from build123d import *

# Parameters (mm, degrees)
SCHIZZO1_R                   = 4.25
SCHIZZO1_R_2                 = 2.75
ESTRUSIONE_ESTRUSIONE1_DEPTH = 2.8
SCHIZZO2_R                   = 4.25
ESTRUSIONE_ESTRUSIONE2_DEPTH = 1
RACCORDO1_R                  = 2


with BuildPart() as part:
    # Schizzo1 → Estrusione-Estrusione1 (new body)
    with BuildSketch(Plane.XY):
        Circle(SCHIZZO1_R)
        Circle(SCHIZZO1_R_2, mode=Mode.SUBTRACT)
    extrude(amount=ESTRUSIONE_ESTRUSIONE1_DEPTH)

    # Schizzo2 → Estrusione-Estrusione2 (add)
    with BuildSketch(Plane.XY.offset(2.8)):
        Circle(SCHIZZO2_R)
    extrude(amount=ESTRUSIONE_ESTRUSIONE2_DEPTH)

    # Raccordo1
    raccordo1_edges = [part.edges().sort_by_distance(p)[0] for p in [
        (-4.25, 0, 3.8),
    ]]
    fillet(raccordo1_edges, radius=RACCORDO1_R)


solid = part.part
Can you work these out from the model? Positions are in its coordinate system, mm. A direction names the side the tool comes from. Coordinates: 2 decimals unless noted, no trailing zeros. Loops run counter-clockwise (first coordinate to the right, second up) from the corner with the lowest first, then second, coordinate; pieces in that order, holes last. Notation, with made-up numbers: (-1.5, 69.5) - (14.5, 69.5) arc R20 ccw to (14.5, 101.5) - close; hole circle Ø7 at (27, -15.5). An arc over 180 degrees is marked (long way). Answer as a JSON object with one key per item and string values. Group by question number.
Item 1: If we section it at C-C (z = 0.9): List the corners of the cut face in (x, y) for me.
Item 2: If we mould it in two halves opening along X, with no side actions, what happens to faces 1 (the face through (-0.596, -2.685, 1.38)), 2 (the face through (0, 0, 3.8)), 3 (the face through (2.285, 3.584, 0.887))? For each: released by +X, released by -X, zero draft, split by the parting line, or undercut.
Item 3: If we section it at D-D (z = 3.4): List the corners of the cut face in (x, y) for me.
Item 4: If we section it at A-A (y = 0): List the corners of the cut face in (x, z) for me.
Item 5: If I drill on L1, parallel to Y at x = 0, z = 1.45; L2, parallel to Y at x = 1, z = 0.2; L3, parallel to X at y = -0.75, z = 0.65, over which ranges is the centre line in solid material (lowest first)? Write a range as from..to.
Item 6: For pin 1 (1.5 mm diameter, centred on y = 3, z = 2.5, fed in from +X); pin 2 (1 mm diameter, centred on x = 1.5, y = -0.5, fed in from -Z); pin 3 (2 mm diameter, centred on y = -1.5, z = 2, fed in from +X), each with a flat end and sliding along its axis, tell me the tip position at first contact or that it passes through.
Item 7: On a 3-axis mill with a long thin cutter (end or side, diameter ignored), from which of +Z, -Z, +X, -X, +Y, -Y can I reach the whole of each face in a straight line? I mean faces 4 (the face through (0, -3, 0)), 5 (the face through (0, 0, 2.8)). Say none if no direction works.
Returned:
{
 "1": {"outline": "circle Ø8.5 at (0, 0); hole circle Ø5.5 at (0, 0)"},
 "2": {"face 1": "undercut", "face 2": "zero draft", "face 3": "split by the parting line"},
 "3": {"outline": "circle Ø6.9 at (0, 0)"},
 "4": {"outline": "(-4.25, 0) - (-2.75, 0) - (-2.75, 2.8) - (2.75, 2.8) - (2.75, 0) - (4.25, 0) - (4.25, 1.8) arc R2 ccw to (2.25, 3.8) - (-2.25, 3.8) arc R2 ccw to (-4.25, 1.8) - close"},
 "5": {"L1": "y = -4.25..-2.75, 2.75..4.25", "L2": "y = -4.13..-2.56, 2.56..4.13", "L3": "x = -4.18..-2.65, 2.65..4.18"},
 "6": {"pin 1": "stops at x = 3.52", "pin 2": "stops at z = 2.8", "pin 3": "stops at x = 4.22"},
 "7": {"face 4": "-Z, +X, -X, +Y, -Y", "face 5": "-Z"}
}
